For this review, take the finished solid that the model builds, in its own axes (mm). Face numbers are marked on the shaded views. A direction names the side the tool comes from. Coordinates: 2 decimals unless noted, no trailing zeros. Write each loop counter-clockwise with the first axis right and the second up, starting at its lowest first coordinate (ties: lowest second). Pieces come first, ordered by that corner, then holes.
```python
from build123d import *

# Parameters (mm, degrees)
CUT_EXTRUDE1_START = 25.4
SKETCH2_R          = 1.5875
CUT_EXTRUDE1_DEPTH = 32.512
CIRPATTERN1_COUNT  = 6
SKETCH3_R          = 3.175
CUT_EXTRUDE2_DEPTH = 50.8
CIRPATTERN2_COUNT  = 6


with BuildPart() as part:
    # Sketch1 → Revolve1 (revolve)
    with BuildSketch(Plane.XY, mode=Mode.PRIVATE) as revolve1_sk:
        Polygon((-12.7, 3.175), (-12.7, 38.1), (-9.525, 38.1), (-9.525, 3.175), (-3.175, 3.175), (-3.175, 50.8), (0, 50.8), (0, 0), (-37.846, 0), (-37.846, 3.175), align=None)
    revolve(revolve1_sk.sketch.rotate(Axis((19.304, 0, 0), (0, 1, 0)), 180), axis=Axis((19.304, 0, 0), (0, 1, 0)))

    # Sketch2 → Cut-Extrude1 (cut)
    with BuildSketch(Plane.XY.offset(CUT_EXTRUDE1_START)):
        with Locations(Location((19.304, 8.255, 0), (0, 0, 180))):
            Circle(SKETCH2_R)
    cut_extrude1 = extrude(amount=CUT_EXTRUDE1_DEPTH, mode=Mode.SUBTRACT)

    # CirPattern1: Cut-Extrude1 ×6 about axis
    cirpattern1_axis = Axis((19.304, 0, 0), (0, -1, 0))
    for i in range(1, CIRPATTERN1_COUNT):
        add(cut_extrude1.rotate(cirpattern1_axis, i * 360 / CIRPATTERN1_COUNT), mode=Mode.SUBTRACT)

    # Sketch3 → Cut-Extrude2 (cut)
    with BuildSketch(Plane(origin=(0, 3.175, 0), x_dir=(1, 0, 0), z_dir=(0, 1, 0))):
        with Locations(Location((-21.940459855, 23.8125, 0), (0, 0, 180))):
            Circle(SKETCH3_R)
    cut_extrude2 = extrude(amount=-CUT_EXTRUDE2_DEPTH, mode=Mode.SUBTRACT)

    # CirPattern2: Cut-Extrude2 ×6 about axis
    cirpattern2_axis = Axis((19.304, 0, 0), (0, 1, 0))
    for i in range(1, CIRPATTERN2_COUNT):
        add(cut_extrude2.rotate(cirpattern2_axis, i * 360 / CIRPATTERN2_COUNT), mode=Mode.SUBTRACT)


solid = part.part
```
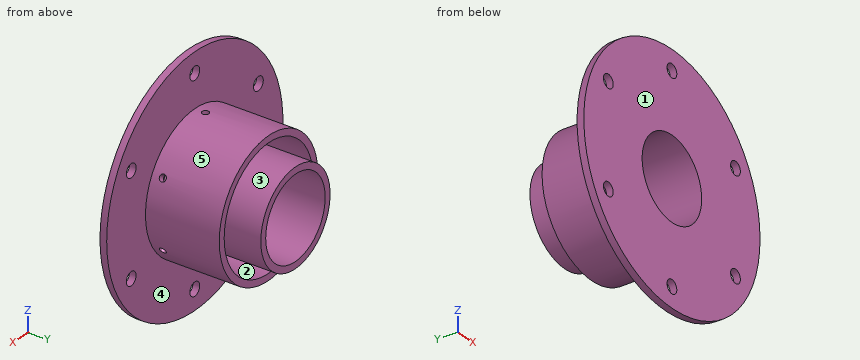
Q1. Clearance check with flat-ended pins moving along their axes: pin 1 Ø3 at (y, z) = (37.5, 12.5) entering from -X; pin 2 Ø10 at (x, z) = (60.55, -23.81) entering from +Y (3 decimals); pin 3 Ø5 at (x, y) = (19.304, 8.255) entering from -Z. State where each tip first meets the part, or that it passes through.
Ans:
pin 1: stops at x = -10.75
pin 2: stops at y = 3.175
pin 3: stops at z = -32
Q2. Tool access review of the marked faces 1 and 2: name each direction out of +Z, -Z, +X, -X, +Y, -Y from which nothing blocks a thin tool from reaching the whole face with its end or side.
Ans:
face 1: +Z, -Z, +X, -X, -Y
face 2: +Y
Q3. Add section B-B (y = 19.5). State the section outline as (x, z) points.
Ans:
outline: circle Ø64.01 at (19.3, 0); circle Ø44.96 at (19.3, 0); hole circle Ø57.66 at (19.3, 0); hole circle Ø38.61 at (19.3, 0)
Q4. For probe 1 along Z at (x, y) = (24.5, 7.5); probe 2 along X at (y, z) = (30, -5); probe 3 along Y at (x, z) = (-29.5, 18.5) (3 decimals), list the stretches that pass through material, from the lowest coordinate up.
Ans:
probe 1: z = -31.58 to -28.36, -21.87 to -18.59, 18.59 to 21.87, 28.36 to 31.58
probe 2: x = -12.31 to -9.09, -2.61 to 0.66, 37.95 to 41.22, 47.7 to 50.92
probe 3: y = 0 to 3.175
Q5. Add section A-A (z = 0). State the section outline as (x, y) points (3 decimals), then the cut area to 3 significant figures.
Ans:
outline: (-37.846, 0) - (0, 0) - (0, 50.8) - (-3.175, 50.8) - (-3.175, 3.175) - (-9.525, 3.175) - (-9.525, 38.1) - (-12.7, 38.1) - (-12.7, 3.175) - (-37.846, 3.175) - close; (38.608, 0) - (76.454, 0) - (76.454, 3.175) - (51.308, 3.175) - (51.308, 38.1) - (48.133, 38.1) - (48.133, 3.175) - (41.783, 3.175) - (41.783, 50.8) - (38.608, 50.8) - close
area: 765 mm2
Q6. Add section D-D (z = -38). State the section outline as (x, y) points (3 decimals), then the cut area to 3 significant figures.
Ans:
outline: (-23.382, 0) - (61.99, 0) - (61.99, 3.175) - (-23.382, 3.175) - close
area: 271 mm2
Q7. Draft analysis for pull direction X (two halves, no side actions). For the marked faces 3, 4 and 5, state which applies: +X half, -X half, draft (parallel to the pull), parting line (faces both ways), or undercut.
Ans:
face 3: undercut
face 4: draft
face 5: parting line
Q8. Add section C-C (y = 47). State the section outline as (x, z) points, then the cut area to 3 significant figures.
Ans:
outline: circle Ø44.96 at (19.3, 0); hole circle Ø38.61 at (19.3, 0)
area: 417 mm2
